Input: dimensioned drawing with shaded views. Units: mm. Origin: part minimum x, y, z. Round coordinates to 2 decimals unless told otherwise and drop trailing zeros. Loops run counter-clockwise (first coordinate to the right, second up) from the corner with the lowest first, then second, coordinate; pieces in that order, holes last. Notation, with made-up numbers: (-6.5, 62) -> (41.5, 62) arc R31 cw to (41.5, 98) -> close; hole circle Ø9 at (58.25, 71). An arc over 180 degrees is marked (long way). Answer as a JSON object with one key per item and string values.
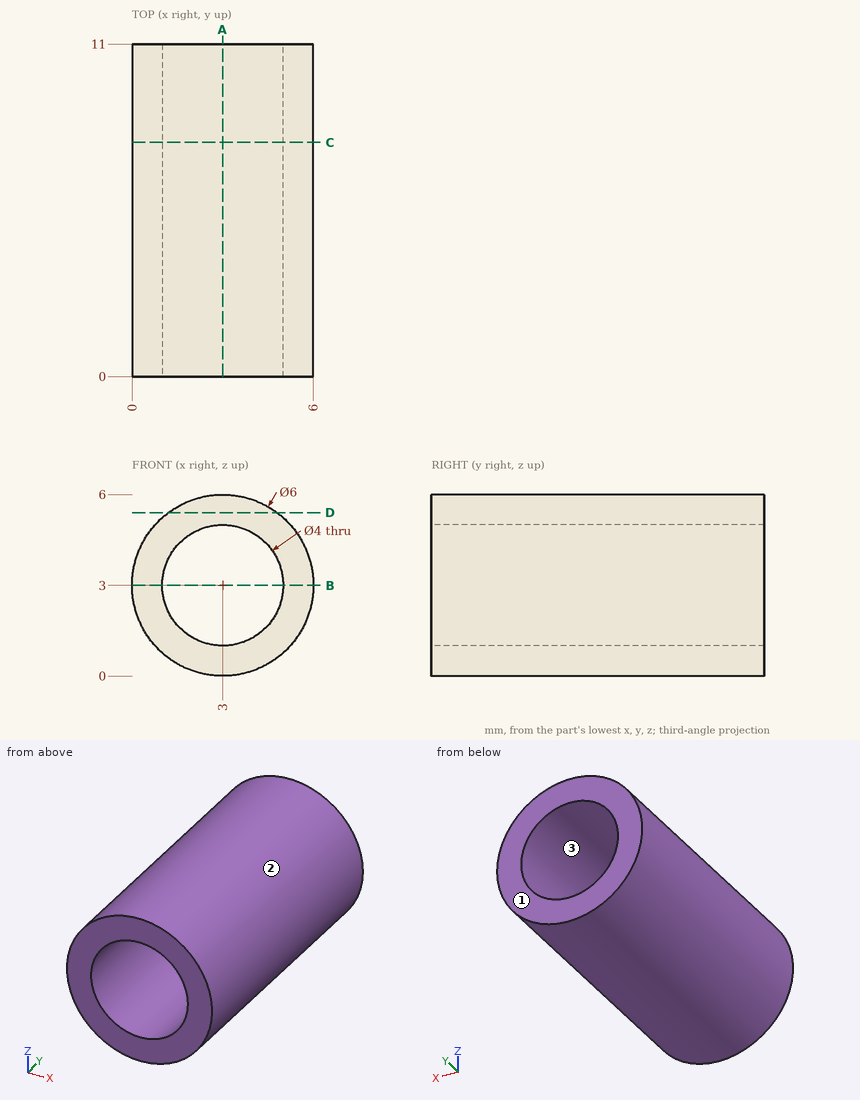
1) Section D-D, the plane z = 5.4. Output: boundary loops of the cut face in (x, y), plus the area to 3 significant figures.
Output:
{"outline": "(1.2, 0) -> (4.8, 0) -> (4.8, 11) -> (1.2, 11) -> close", "area": "39.6 mm^2"}
2) Section C-C, the plane y = 7.75. Output: boundary loops of the cut face in (x, z).
Output:
{"outline": "circle Ø6 at (3, 3); hole circle Ø4 at (3, 3)"}
3) Draft query along X for the marked faces 1, 2 and 3. Return one class per face: +X half, -X half, draft (parallel to the pull), parting line (faces both ways), or undercut.
Output:
{"face 1": "draft", "face 2": "parting line", "face 3": "undercut"}
4) Section B-B, the plane z = 3. Output: boundary loops of the cut face in (x, y), plus the area to 3 significant figures.
Output:
{"outline": "(0, 0) -> (1, 0) -> (1, 11) -> (0, 11) -> close; (5, 0) -> (6, 0) -> (6, 11) -> (5, 11) -> close", "area": "22.0 mm^2"}
5) Ray query, probe 1 along Z at (x, y) = (3, 7); probe 2 along Z at (x, y) = (2.3, 8.5). Return the intervals inside material, ascending.
Output:
{"probe 1": "z = 0 to 1, 5 to 6", "probe 2": "z = 0.08 to 1.13, 4.87 to 5.92"}
6) Contact query for flat-ended pins moving along their axis: P1, Ø1.5, axis at x = 1, y = 10, coming from the -Z side; P2, Ø1, axis at x = 5.5, y = 3.5, coming from the -Z side; P3, Ø1.5, axis at x = 2, y = 8, coming from the +Z side; P4, Ø2.5, axis at x = 3, z = 3, coming from the +Y side. Output: stop coordinate, or through.
Output:
{"P1": "stops at z = 0.27", "P2": "stops at z = 0.76", "P3": "stops at z = 5.99", "P4": "passes through"}
7) Section A-A, the plane x = 3. Output: boundary loops of the cut face in (y, z), plus the area to 3 significant figures.
Output:
{"outline": "(0, 0) -> (11, 0) -> (11, 1) -> (0, 1) -> close; (0, 5) -> (11, 5) -> (11, 6) -> (0, 6) -> close", "area": "22.0 mm^2"}
